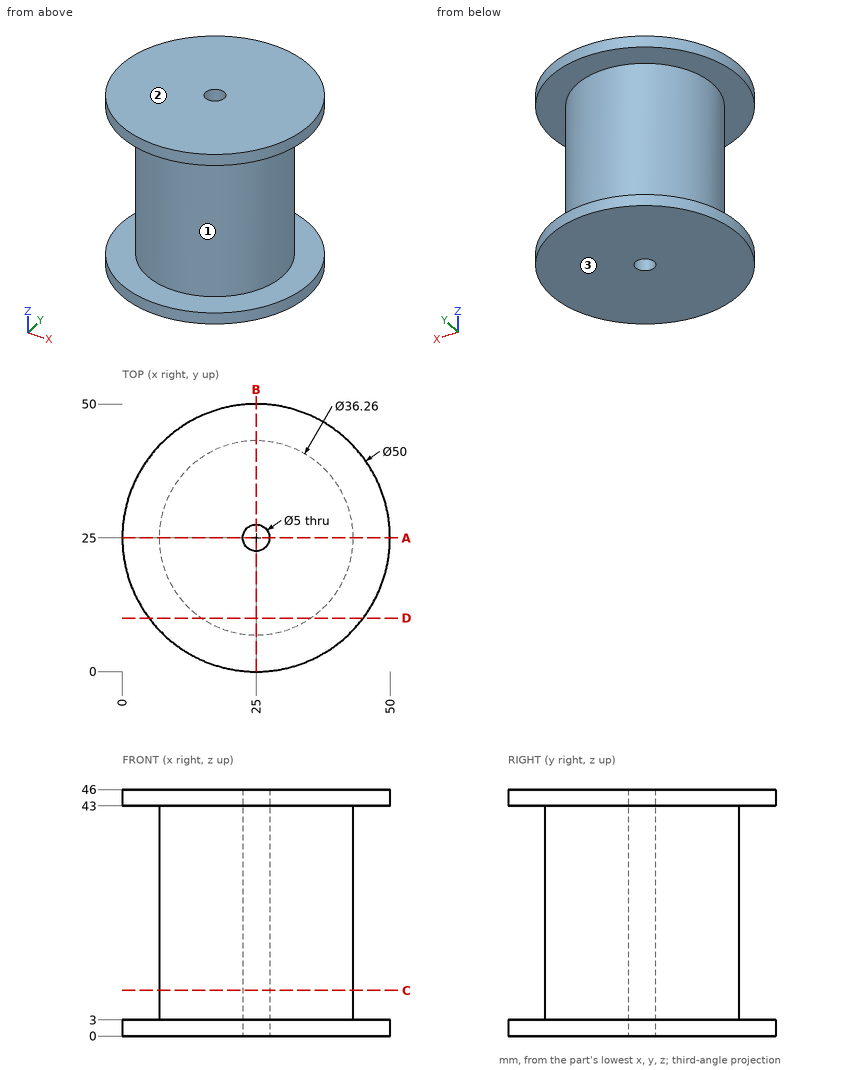
Study the drawing (mm; zero at the part's minimum x, y, z) and answer. Give positions to 0.01 mm unless a question says otherwise; leave off trailing zeros. Loops run counter-clockwise (first coordinate to the right, second up) from the corner with the lowest first, then second, coordinate; pieces in that order, holes last. Notation, with made-up numbers: (17, 73.25) -> (37, 73.25) arc R16 ccw to (37, 98.25) -> close; hole circle Ø5 at (-40, -23.5). An arc over 180 degrees is marked (long way). Write item = value, one per line. Start each with the question number.
(1) The mould has two halves that part along Z. Classify the marked faces 1, 2 and 3: +Z half, -Z half, draft (parallel to the pull), parting line (faces both ways), or undercut.
(2) Find section C-C on z = 8.5. Give the vertices of the cut face in (x, y), and give its area (3 significant figures).
(3) Find the intervals of material crossed by probe 1 along Y at (x, z) = (25, 21); probe 2 along Z at (x, y) = (43.5, 28); probe 3 along X at (y, z) = (26.5, 19), in increasing order. Write a range as from..to.
(4) Given pin 1 Ø2 at (x, z) = (12, 14) entering from -Y; pin 2 Ø8 at (x, z) = (11, 31.5) entering from -Y; pin 3 Ø10 at (x, z) = (26.5, 26.5) entering from -Y; pin 4 Ø3 at (x, y) = (25, 25) entering from -Z, each flat-ended and moving along its own axis, determine where each tip first touches the part or whether it passes through.
(5) Find section D-D on y = 10. Give the vertices of the cut face in (x, z), and give its area (3 significant figures).
(6) Find section A-A on y = 25. Give the vertices of the cut face in (x, z), and give its area (3 significant figures).
From the geometry:
q1.face_1 = undercut
q1.face_2 = +Z half
q1.face_3 = -Z half
q2.outline = circle Ø36.26 at (25, 25); hole circle Ø5 at (25, 25)
q2.area = 1,010 mm^2
q3.probe_1 = 6.87..22.5, 27.5..43.13
q3.probe_2 = 0..3, 43..46
q3.probe_3 = 6.93..23, 27..43.07
q4.pin_1 = 11.41
q4.pin_2 = 9.88
q4.pin_3 = 6.87
q4.pin_4 = through
q5.outline = (5, 0) -> (45, 0) -> (45, 3) -> (35.18, 3) -> (35.18, 43) -> (45, 43) -> (45, 46) -> (5, 46) -> (5, 43) -> (14.82, 43) -> (14.82, 3) -> (5, 3) -> close
q5.area = 1,050 mm^2
q6.outline = (0, 0) -> (22.5, 0) -> (22.5, 46) -> (0, 46) -> (0, 43) -> (6.87, 43) -> (6.87, 3) -> (0, 3) -> close; (27.5, 0) -> (50, 0) -> (50, 3) -> (43.13, 3) -> (43.13, 43) -> (50, 43) -> (50, 46) -> (27.5, 46) -> close
q6.area = 1,520 mm^2
